```python
from build123d import *

# Parameters (mm, degrees)
F0_W            = 300
F0_H            = 300
F1_DEPTH        = 6
F2_W            = 150
F2_H            = 6
F3_DEPTH        = 6
F3_COPIES_COUNT = 4
F5_W            = 6
F5_H            = 150
F6_DEPTH        = 6


# Not quite as in the source:
# - a pattern or mirror of a feature is missing from the dataset's text; its kind, count and spacing are read off the source's solid


with BuildPart() as f1:
    # F0 (on Top) → F1 (new body)
    with BuildSketch(Plane.XY):
        Rectangle(F0_W, F0_H)
    extrude(amount=F1_DEPTH)

    # F2 (on face) → F3 (cut, through all)
    with BuildSketch(Plane.XY.offset(6)):
        with Locations((0, -147)):
            Rectangle(F2_W, F2_H)
    f3 = extrude(amount=-F3_DEPTH, mode=Mode.SUBTRACT)

    # F3_copies: F3 ×4 about axis
    f3_copies_axis = Axis((0, 0, 0), (0, 0, 1))
    for i in range(1, F3_COPIES_COUNT):
        add(f3.rotate(f3_copies_axis, i * 360 / F3_COPIES_COUNT), mode=Mode.SUBTRACT)

    # F5 (on face) → F6 (cut, through all)
    with BuildSketch(Plane.XY.offset(6)):
        with Locations((-50, 0)):
            Rectangle(F5_W, F5_H)
        with Locations((50, 0)):
            Rectangle(F5_W, F5_H)
    extrude(amount=-F6_DEPTH, mode=Mode.SUBTRACT)


solid = f1.part
```
Verification items for the finished model (mm, model axes). Give positions to 0.01 mm unless a question says otherwise; leave off trailing zeros. Order: outer loops, then holes, each group sorted by start corner. A loop starts at its lowest first (then second) coordinate and runs counter-clockwise, first axis right, second up. Notation, with made-up numbers: (10, -14.75) - (18, -14.75) arc R20 cw to (18, -2.75) - close; hole circle Ø8 at (8, 50). An arc over 180 degrees is marked (long way). Answer as CSV lines item,"result". Start each with the question number.
Item 1: Gauge pin test, flat ends, axial feed: pin 1 (1.8 mm diameter, centred on x = 34.5, z = 2.5, fed in from -Y); pin 2 (3 mm diameter, centred on x = -20.5, z = 3.5, fed in from +Y). Record the tip position at first contact, or that the pin passes through.
Item 2: Section check A-A, the plane y = 9.5. Record the boundary of the cut face in (x, z).
Item 3: Section check C-C, the plane x = 65.5. Record the boundary of the cut face in (y, z), plus the area to 3 significant figures.
Item 4: Section check B-B, the plane z = 3.95. Record the boundary of the cut face in (x, y).
Item 5: Material ranges on L1, parallel to X at y = 28, z = 2.4; L2, parallel to Y at x = -52, z = 5.3; L3, parallel to Y at x = 16.5, z = 3, recorded low to high.
Filled in:
1,pin 1,"y = -144"
1,pin 2,"y = 144"
2,outline,"(-144, 0) - (-53, 0) - (-53, 6) - (-144, 6) - close; (-47, 0) - (47, 0) - (47, 6) - (-47, 6) - close; (53, 0) - (144, 0) - (144, 6) - (53, 6) - close"
3,outline,"(-144, 0) - (144, 0) - (144, 6) - (-144, 6) - close"
3,area,"1,730 mm^2"
4,outline,"(-150, -150) - (-75, -150) - (-75, -144) - (75, -144) - (75, -150) - (150, -150) - (150, -75) - (144, -75) - (144, 75) - (150, 75) - (150, 150) - (75, 150) - (75, 144) - (-75, 144) - (-75, 150) - (-150, 150) - (-150, 75) - (-144, 75) - (-144, -75) - (-150, -75) - close; hole (-53, -75) - (-47, -75) - (-47, 75) - (-53, 75) - close; hole (47, -75) - (53, -75) - (53, 75) - (47, 75) - close"
5,L1,"-144 to -53, -47 to 47, 53 to 144"
5,L2,"-144 to -75, 75 to 144"
5,L3,"-144 to 144"
